The figure shows three views and two pictorial views of one solid part (mm, origin at its lowest corner). Answer the questions. Round coordinates to 2 decimals unless told otherwise and drop trailing zeros. Write each loop counter-clockwise with the first axis right and the second up, starting at its lowest first coordinate (ties: lowest second). Pieces come first, ordered by that corner, then holes. Notation, with made-up numbers: M 53,36 L 90,36 A7 ccw 90,43 Z; hole C -12.75,32.5 d6. An arc over 180 degrees is marked long. Use one line per item in the form item = value. Start each with the question number.
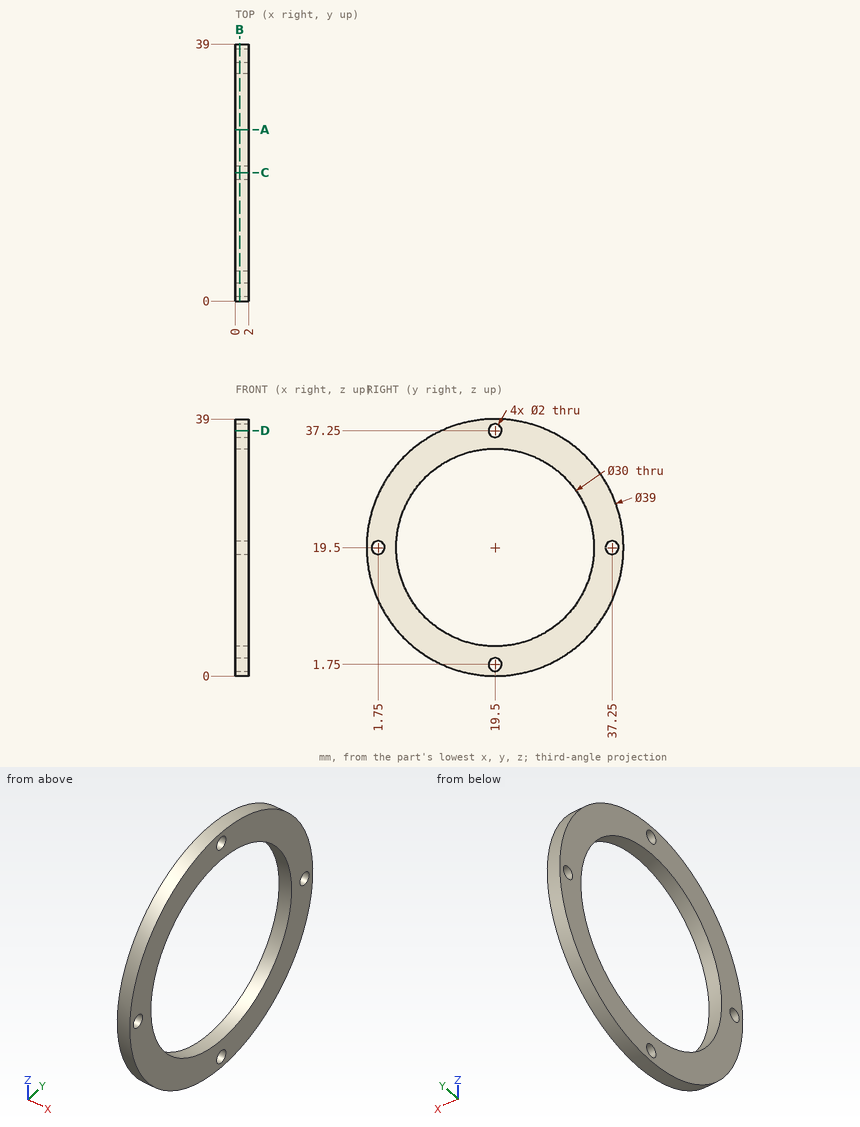
Q1. Find section B-B on x = 0.65. Write down the section's boundary in (y, z), and give its area (3 significant figures).
Q2. Straight lines are drawn through the part: line 1 (Y direction, x = 0.65, z = 19.5); line 2 (Y direction, x = 0.4, z = 1.75); line 3 (Z direction, x = 0.8, y = 32). For each, find the intervals that lie inside material, in ascending order. Write a range as [from, to].
Q3. Find section D-D on z = 37.25. Write down the section's boundary in (x, y).
Q4. Find section A-A on y = 26. Write down the section's boundary in (x, z).
Q5. Find section C-C on y = 19.5. Write down the section's boundary in (x, z).
Response:
q1.outline = C 19.5,19.5 d39; hole C 1.75,19.5 d2; hole C 19.5,19.5 d30; hole C 19.5,1.75 d2; hole C 19.5,37.25 d2; hole C 37.25,19.5 d2
q1.area = 475 mm²
q2.line_1 = [0, 0.75], [2.75, 4.5], [34.5, 36.25], [38.25, 39]
q2.line_2 = [11.43, 18.5], [20.5, 27.57]
q2.line_3 = [4.53, 11.21], [27.79, 34.47]
q3.outline = M 0,11.43 L 2,11.43 L 2,18.5 L 0,18.5 Z; M 0,20.5 L 2,20.5 L 2,27.57 L 0,27.57 Z
q4.outline = M 0,1.12 L 2,1.12 L 2,5.98 L 0,5.98 Z; M 0,33.02 L 2,33.02 L 2,37.88 L 0,37.88 Z
q5.outline = M 0,0 L 2,0 L 2,0.75 L 0,0.75 Z; M 0,2.75 L 2,2.75 L 2,4.5 L 0,4.5 Z; M 0,34.5 L 2,34.5 L 2,36.25 L 0,36.25 Z; M 0,38.25 L 2,38.25 L 2,39 L 0,39 Z
